Build history of the part. All positions in model axes, mm. A direction names the side the tool comes from. Coordinates: 2 decimals unless noted, no trailing zeros. Order: outer loops, then holes, each group sorted by start corner. A loop starts at its lowest first (then second) coordinate and runs counter-clockwise, first axis right, second up. Notation, with made-up numbers: (47, -16) - (75, -16) arc R8 cw to (75, -3) - close; hole circle Ø8 at (-33, 88). An arc over 180 degrees is marked (long way). Answer as CSV lines item,"result". Start each with the question number.
from build123d import *

# Parameters (mm, degrees)
SKETCH_1_W          = 113
SKETCH_1_H          = 76
SKETCH_1_W_2        = 107
SKETCH_1_H_2        = 70
EXTRUDE_1_DEPTH     = 40
SKETCH_2_W          = 113
SKETCH_2_H          = 76
EXTRUDE_2_DEPTH     = 2
SKETCH_3_R          = 1.05
CUT_EXTRUDE_1_DEPTH = 127.400158228
SKETCH_6_W          = 60
SKETCH_6_H          = 30
CUT_EXTRUDE_2_DEPTH = 102.416221582
SKETCH_7_W          = 107
SKETCH_7_H          = 8.791278805
CUT_EXTRUDE_3_DEPTH = 102.416221582
SKETCH_9_W          = 26.200451213
SKETCH_9_H          = 60
CUT_EXTRUDE_4_DEPTH = 3
SKETCH_10_W         = 30
SKETCH_10_H         = 50
CUT_EXTRUDE_5_DEPTH = 3
SKETCH_13_W         = 107
SKETCH_13_H         = 40
CUT_EXTRUDE_6_DEPTH = 3
SKETCH_17_W         = 113
SKETCH_17_H         = 76
EXTRUDE_4_DEPTH     = 1
SKETCH_18_W         = 107
SKETCH_18_H         = 3
CUT_EXTRUDE_7_DEPTH = 2
FILLET_1_R          = 2
SKETCH_19_R         = 1.15
CUT_EXTRUDE_8_DEPTH = 127.400158228


with BuildPart() as part:
    # 草图1 → 凸台-拉伸1 (new body)
    with BuildSketch(Plane.XY):
        Rectangle(SKETCH_1_W, SKETCH_1_H)
        Rectangle(SKETCH_1_W_2, SKETCH_1_H_2, mode=Mode.SUBTRACT)
    extrude(amount=EXTRUDE_1_DEPTH)

    # 草图2 → 凸台-拉伸2 (add)
    with BuildSketch(Plane.XY.offset(40)):
        Rectangle(SKETCH_2_W, SKETCH_2_H)
    extrude(amount=EXTRUDE_2_DEPTH)

    # 草图3 → 切除-拉伸1 (cut, through all)
    with BuildSketch(Plane.ZY.offset(56.5)):
        with Locations((5, 20)):
            Circle(SKETCH_3_R)
        with Locations(Location((5, -20, 0), (0, 0, 180))):
            Circle(SKETCH_3_R)
    extrude(amount=-CUT_EXTRUDE_1_DEPTH, mode=Mode.SUBTRACT)

    # 草图6 → 切除-拉伸2 (cut, through all)
    with BuildSketch(Plane.XZ.offset(-35)):
        with Locations((-23.5, 15)):
            Rectangle(SKETCH_6_W, SKETCH_6_H)
    extrude(amount=-CUT_EXTRUDE_2_DEPTH, mode=Mode.SUBTRACT)

    # 草图7 → 切除-拉伸3 (cut, through all)
    with BuildSketch(Plane(origin=(0, -35, 0), x_dir=(1, 0, 0), z_dir=(0, 1, 0))):
        with Locations((0, -4.395639403)):
            Rectangle(SKETCH_7_W, SKETCH_7_H)
    extrude(amount=-CUT_EXTRUDE_3_DEPTH, mode=Mode.SUBTRACT)

    # 草图9 → 切除-拉伸4 (cut)
    with BuildSketch(Plane(origin=(56.5, 0, 0), x_dir=(0, 0, -1), z_dir=(1, 0, 0))):
        with Locations((-23.100225607, 0)):
            Rectangle(SKETCH_9_W, SKETCH_9_H)
    extrude(amount=-CUT_EXTRUDE_4_DEPTH, mode=Mode.SUBTRACT)

    # 草图10 → 切除-拉伸5 (cut)
    with BuildSketch(Plane.ZY.offset(56.5)):
        with Locations((25, 0)):
            Rectangle(SKETCH_10_W, SKETCH_10_H)
    extrude(amount=-CUT_EXTRUDE_5_DEPTH, mode=Mode.SUBTRACT)

    # 草图13 → 切除-拉伸6 (cut)
    with BuildSketch(Plane(origin=(0, 38, 0), x_dir=(1, 0, 0), z_dir=(0, 1, 0))):
        with Locations((0, -20)):
            Rectangle(SKETCH_13_W, SKETCH_13_H)
    extrude(amount=-CUT_EXTRUDE_6_DEPTH, mode=Mode.SUBTRACT)

    # 草图17 → 凸台-拉伸4 (add)
    with BuildSketch(Plane(origin=(0, 0, 40), x_dir=(-1, 0, 0), z_dir=(0, 0, -1))):
        Rectangle(SKETCH_17_W, SKETCH_17_H)
    extrude(amount=EXTRUDE_4_DEPTH)

    # 草图18 → 切除-拉伸7 (cut)
    with BuildSketch(Plane(origin=(0, 0, 8.791278805), x_dir=(-1, 0, 0), z_dir=(0, 0, -1))):
        with Locations((0, -36.5)):
            Rectangle(SKETCH_18_W, SKETCH_18_H)
    extrude(amount=-CUT_EXTRUDE_7_DEPTH, mode=Mode.SUBTRACT)

    # 圆角1
    fillet_1_edges = [part.edges().sort_by_distance(p)[0] for p in [
        (-55, -25, 10),
        (-55, 25, 10),
        (-55, 25, 39),
        (-55, -25, 39),
        (0, -38, 42),
        (0, 38, 42),
        (-56.5, 38, 21),
        (56.5, 38, 21),
        (56.5, -38, 21),
        (-56.5, -38, 21),
        (55, 30, 36.200451213),
        (55, 30, 10),
        (55, -30, 10),
        (55, -30, 36.200451213),
    ]]
    fillet(fillet_1_edges, radius=FILLET_1_R)

    # 草图19 → 切除-拉伸8 (cut, through all)
    with BuildSketch(Plane(origin=(56.5, 0, 0), x_dir=(0, 0, -1), z_dir=(1, 0, 0))):
        with Locations((-5, 20)):
            Circle(SKETCH_19_R)
        with Locations((-5, -20)):
            Circle(SKETCH_19_R)
    extrude(amount=-CUT_EXTRUDE_8_DEPTH, mode=Mode.SUBTRACT)


solid = part.part
(1) Drop flat-ended pins along their axis: pin 1 Ø14 at (x, z) = (-1, 20.5) entering from +Y; pin 2 Ø1.5 at (x, y) = (-23.5, -14) entering from -Z; pin 3 Ø0.9 at (x, y) = (19.5, -36) entering from -Z. Give the stop position or say it passes through.
(2) Band-saw the part on B-B on z = 5. List the corners of the cut face in (x, y), plus the area to 3 significant figures.
(3) Band-saw the part on C-C on z = 26. List the corners of the cut face in (x, y).
(4) Which spindle directions (+Z, -Z, +X, -X, +Y, -Y) get a long thin tool onto all of the face, cutting with end or side? Do faces 1 (the flat face through (53.5, 1, 7)), 2 (the flat face through (1, -36, 10.791)), 3 (the flat face through (-55, 0, 10)). Say none if no direction does.
(5) Band-saw the part on D-D on y = 20. List the corners of the cut face in (x, z).
(6) Band-saw the part on A-A on y = 8. List the corners of the cut face in (x, z).
(7) Probe L1, parallel to Y at x = -54.25, z = 5; L2, parallel to X at y = 31.5, z = 16.5; L3, parallel to Y at x = 55.6, z = 5. List the from-to ranges inside material, lowest first. Write a range as [from, to].
(8) Pull direction X, two halves, no side cores. Call faces 4 (the flat face through (-1, 1, 42)), 5 (the flat face through (-1, -35, 25)), 6 (the flat face through (-56.5, -1, 7)): +X half, -X half, draft (parallel to the pull), parting line (faces both ways), or undercut.
Filled in:
1,pin 1,"stops at y = -35"
1,pin 2,"stops at z = 39"
1,pin 3,"stops at z = 10.79"
2,outline,"(-56.5, -36) arc R2 ccw to (-54.5, -38) - (-53.5, -38) - (-53.5, -21.15) - (-56.5, -21.15) - close; (-56.5, -18.85) - (-53.5, -18.85) - (-53.5, 18.85) - (-56.5, 18.85) - close; (-56.5, 21.15) - (-53.5, 21.15) - (-53.5, 38) - (-54.5, 38) arc R2 ccw to (-56.5, 36) - close; (53.5, -38) - (54.5, -38) arc R2 ccw to (56.5, -36) - (56.5, -21.15) - (53.5, -21.15) - close; (53.5, -18.85) - (56.5, -18.85) - (56.5, 18.85) - (53.5, 18.85) - close; (53.5, 21.15) - (56.5, 21.15) - (56.5, 36) arc R2 ccw to (54.5, 38) - (53.5, 38) - close"
2,area,"425 mm^2"
3,outline,"(-56.5, -36) arc R2 ccw to (-54.5, -38) - (54.5, -38) arc R2 ccw to (56.5, -36) - (56.5, -30) - (53.5, -30) - (53.5, -35) - (-53.5, -35) - (-53.5, -25) - (-56.5, -25) - close; (-56.5, 25) - (-53.5, 25) - (-53.5, 38) - (-54.5, 38) arc R2 ccw to (-56.5, 36) - close; (53.5, 30) - (56.5, 30) - (56.5, 36) arc R2 ccw to (54.5, 38) - (53.5, 38) - close"
4,face 1,"-Z, +Y"
4,face 2,"-Z, +Y, -Y"
4,face 3,"+X, -X"
5,outline,"(-56.5, 0) - (-53.5, 0) - (-53.5, 3.85) - (-56.5, 3.85) - close; (-56.5, 6.15) - (-53.5, 6.15) - (-53.5, 10) - (-56.5, 10) - close; (-56.5, 39) - (53.5, 39) - (53.5, 36.2) - (56.5, 36.2) - (56.5, 42) - (-56.5, 42) - close; (53.5, 0) - (56.5, 0) - (56.5, 3.85) - (53.5, 3.85) - close; (53.5, 6.15) - (56.5, 6.15) - (56.5, 10) - (53.5, 10) - close"
6,outline,"(-56.5, 0) - (-53.5, 0) - (-53.5, 10) - (-56.5, 10) - close; (-56.5, 39) - (53.5, 39) - (53.5, 36.2) - (56.5, 36.2) - (56.5, 42) - (-56.5, 42) - close; (53.5, 0) - (56.5, 0) - (56.5, 10) - (53.5, 10) - close"
7,L1,"y = [-38, -21.15], [-18.85, 18.85], [21.15, 38]"
7,L2,"x = [-56.5, -53.5], [53.5, 56.5]"
7,L3,"y = [-37.67, -21.15], [-18.85, 18.85], [21.15, 37.67]"
8,face 4,"draft"
8,face 5,"undercut"
8,face 6,"-X half"
